Autodesk Inventor part; units mm, degrees
ref_plane "Work Plane1" through (0, 18, 0) normal (0, 1, 0) x (-1, 0, 0)
ref_plane "YZ Plane" through (0, 0, 0) normal (1, 0, 0) x (0, 1, 0)
ref_plane "XY Plane" through (0, 0, 0) normal (0, 0, 1) x (1, 0, 0)
sketch "Sketch1" plane through (0, 0, 0) normal (0, 1, 0) x (-1, 0, 0)
  line L0 (0, 0) -> (80, 0) construction
  line L1 (80, 0) -> (80, 30) construction
  line L2 (80, 30) -> (0, 30) construction
  line L3 (0, 30) -> (0, 0) construction
  dimension "d0" = 80
  dimension "d1" = 30
sketch "Sketch2" plane through (0, 0, 0) normal (0, 1, 0) x (-1, 0, 0)
  line L0 (80, 0) -> (69, 0)
  line L1 (69, 0) -> (69, 30)
  line L2 (69, 30) -> (80, 30)
  line L3 (80, 30) -> (80, 0)
  line L4 (0, 0) -> (11, 0)
  line L5 (11, 0) -> (11, 30)
  line L6 (11, 30) -> (0, 30)
  line L7 (0, 30) -> (0, 0)
  line L8 (57, 0) -> (46, 0)
  line L9 (46, 0) -> (46, 30)
  line L10 (46, 30) -> (57, 30)
  line L11 (57, 30) -> (57, 0)
  line L12 (34, 0) -> (23, 0)
  line L13 (23, 0) -> (23, 30)
  line L14 (23, 30) -> (34, 30)
  line L15 (34, 30) -> (34, 0)
  line L16 (69, 15) -> (57, 15) construction
  line L17 (46, 15) -> (34, 15) construction
  line L18 (23, 15) -> (11, 15) construction
  line L19 (72, 3) -> (77, 3)
  line L20 (77, 3) -> (77, 27)
  line L21 (77, 27) -> (72, 27)
  line L22 (72, 27) -> (72, 3)
  line L23 (54, 3) -> (49, 3)
  line L24 (49, 3) -> (49, 27)
  line L25 (49, 27) -> (54, 27)
  line L26 (54, 27) -> (54, 3)
  line L27 (31, 3) -> (26, 3)
  line L28 (26, 3) -> (26, 27)
  line L29 (26, 27) -> (31, 27)
  line L30 (31, 27) -> (31, 3)
  line L31 (8, 27) -> (8, 3)
  line L32 (8, 3) -> (3, 3)
  line L33 (3, 3) -> (3, 27)
  line L34 (3, 27) -> (8, 27)
  dimension "d2" = 11
  dimension "d3" = 30
  dimension "d4" = 11
  dimension "d6" = 11
  dimension "d8" = 11
  dimension "d9" = 80
  dimension "d10" = 3
  dimension "d11" = 3
  dimension "d12" = 3
  dimension "d13" = 3
extrude "Extrusion1" add sketch "Sketch2" along normal blind 15
sketch "Sketch3" plane through (0, 15, 0) normal (0, 1, 0) x (1, 0, 0)
  line L0 (-69, 0) -> (-80, 0)
  line L1 (-80, 0) -> (-69, 0)
  line L2 (-69, 0) -> (-69, -30)
  line L3 (-69, -30) -> (-80, -30)
  line L4 (-80, -30) -> (-80, 0)
  line L5 (-57, 0) -> (-46, 0)
  line L6 (-46, 0) -> (-46, -30)
  line L7 (-46, -30) -> (-57, -30)
  line L8 (-57, -30) -> (-57, 0)
  line L9 (-34, 0) -> (-23, 0)
  line L10 (-23, 0) -> (-23, -30)
  line L11 (-23, -30) -> (-34, -30)
  line L12 (-34, -30) -> (-34, 0)
  line L13 (-11, 0) -> (0, 0)
  line L14 (0, 0) -> (0, -30)
  line L15 (0, -30) -> (-11, -30)
  line L16 (-11, -30) -> (-11, 0)
  dimension "d16" = 30
  dimension "d19" = 23
extrude "Extrusion2" add sketch "Sketch3" along normal blind 3
sketch "Sketch4" plane through (-69, 0, 30) normal (1, 0, 0) x (0, 0, -1)
  circle A0 centre (7.5, 8) radius 1.5
  line L0 (3, 0) -> (27, 0)
  line L1 (0, 0) -> (0, 18) construction
  dimension "d26" = 3
  dimension "d28" = 8
  dimension "d29" = 7.5
extrude "Extrusion3" cut sketch "Sketch4" against normal blind 3
sketch "Sketch5" plane through (-57, 0, 0) normal (-1, 0, 0) x (0, 0, 1)
  circle A0 centre (22.5, 8) radius 1.5
  line L0 (30, 0) -> (30, 18)
  line L1 (3, 0) -> (27, 0)
  point P0 (0, 0)
  dimension "d33" = 3
  dimension "d34" = 7.5
  dimension "d35" = 8
extrude "Extrusion4" cut sketch "Sketch5" against normal blind 3
sketch "Sketch6" plane through (-46, 0, 30) normal (1, 0, 0) x (0, 0, -1)
  circle A0 centre (22.5, 8) radius 1.5
  line L0 (30, 0) -> (30, 18)
  line L1 (3, 0) -> (27, 0)
  dimension "d38" = 3
  dimension "d39" = 7.5
  dimension "d40" = 8
sketch "Sketch7" plane through (-34, 0, 0) normal (-1, 0, 0) x (0, 0, 1)
  circle A0 centre (7.5, 8) radius 1.5
  line L0 (3, 0) -> (27, 0)
  line L1 (0, 0) -> (0, 18)
  dimension "d41" = 3
  dimension "d42" = 8
  dimension "d43" = 7.5
sketch "Sketch8" plane through (-23, 0, 30) normal (1, 0, 0) x (0, 0, -1)
  circle A0 centre (7.5, 8) radius 1.5
  line L0 (3, 0) -> (27, 0)
  line L1 (0, 0) -> (0, 18)
  point P0 (30, 0)
  dimension "d44" = 3
  dimension "d45" = 8
  dimension "d46" = 7.5
sketch "Sketch9" plane through (-11, 0, 0) normal (-1, 0, 0) x (0, 0, 1)
  point P0 (0, 0)
sketch "Sketch10" plane through (-11, 0, 0) normal (-1, 0, 0) x (0, 0, 1)
  circle A0 centre (22.5, 8) radius 1.5
  line L0 (30, 0) -> (30, 18)
  line L1 (3, 0) -> (27, 0)
  point P0 (0, 0)
  dimension "d47" = 3
  dimension "d48" = 7.5
  dimension "d49" = 8
extrude "Extrusion5" cut sketch "Sketch6" against normal blind 3
extrude "Extrusion6" cut sketch "Sketch7" against normal blind 3
extrude "Extrusion7" cut sketch "Sketch8" against normal blind 3
extrude "Extrusion8" cut sketch "Sketch10" against normal blind 3
ref_plane "Work Plane1" through (0, 18, 0) normal (0, 1, 0) x (-1, 0, 0)
sketch "Sketch12" plane through (0, 18, 0) normal (0, 1, 0) x (-1, 0, 0)
  line L0 (80, 30) -> (50, 30)
  line L1 (50, 30) -> (50, 22)
  line L2 (50, 22) -> (80, 22)
  line L3 (80, 22) -> (80, 30)
  line L4 (55, 0) -> (25, 0)
  line L5 (25, 0) -> (25, 8)
  line L6 (25, 8) -> (55, 8)
  line L7 (55, 8) -> (55, 0)
  line L8 (31, 3) -> (31, 27)
  line L9 (31, 22) -> (1, 22)
  line L10 (1, 22) -> (1, 30)
  line L11 (1, 30) -> (31, 30)
  line L12 (31, 30) -> (31, 22)
  point P0 (0, 0)
  dimension "d59" = 30
  dimension "d60" = 8
  dimension "d61" = 30
  dimension "d62" = 8
  dimension "d63" = 30
sketch "Sketch13" plane through (0, 18, 0) normal (0, 1, 0) x (-1, 0, 0)
  line L0 (74.3573, 0) -> (62.3573, 0)
  line L1 (62.3573, 0) -> (62.3573, 15)
  line L2 (62.3573, 15) -> (74.3573, 15)
  line L3 (74.3573, 15) -> (74.3573, 0)
  line L4 (48, 12) -> (36, 12)
  line L5 (36, 12) -> (36, 21)
  line L6 (36, 21) -> (48, 21)
  line L7 (48, 21) -> (48, 12)
  line L8 (0, 0) -> (11, 0)
  line L9 (4, 0) -> (17, 0)
  line L10 (17, 0) -> (17, 17)
  line L11 (17, 17) -> (4, 17)
  line L12 (4, 17) -> (4, 0)
  dimension "d64" = 12
  dimension "d65" = 15
  dimension "d66" = 12
  dimension "d67" = 13
  dimension "d68" = 17
extrude "Extrusion9" add sketch "Sketch13" along normal blind 2
extrude "Extrusion10" add sketch "Sketch12" along normal blind 4
sketch "Sketch14" plane through (0, 20, 0) normal (0, 1, 0) x (1, 0, 0)
  line L0 (-65, -4) -> (-41.7529, -4)
  line L1 (-41.7529, -4) -> (-41.7529, -17.4715)
  line L2 (-41.7529, -17.4715) -> (-65, -17.4715)
  line L3 (-65, -17.4715) -> (-65, -4)
  line L4 (-12, -25) -> (-28.5, -25)
  line L5 (-28.5, -25) -> (-28.5, -4)
  line L6 (-28.5, -4) -> (-12, -4)
  line L7 (-12, -4) -> (-12, -25)
  point P0 (0, 0)
  dimension "d73" = 16.5
extrude "Extrusion11" add sketch "Sketch14" along normal blind 4
sketch "Sketch15" plane through (0, 20, 0) normal (0, 1, 0) x (1, 0, 0)
  line L0 (-69, -30) -> (-69, -22)
  line L1 (-69, -26) -> (-17, -26)
  line L2 (-17, -26) -> (-17, -6)
  line L3 (-17, -6) -> (-69, -6)
  line L4 (-69, -6) -> (-69, -26)
  point P0 (0, 0)
  dimension "d76" = 52
  dimension "d77" = 20
extrude "Extrusion12" add sketch "Sketch15" along normal blind 3
sketch "Sketch16" plane through (0, 0, 0) normal (0, 1, 0) x (-1, 0, 0)
  line L0 (69, 30) -> (80, 30)
  line L1 (80, 30) -> (80, 36)
  line L2 (69, 30) -> (69, 36)
  line L3 (69, 36) -> (74.8182, 41.4908)
  line L4 (74.8182, 41.4908) -> (80, 36)
  circle A0 centre (74.5, 36) radius 1.25
  line L5 (74.5, 36) -> (80, 36) construction
  line L6 (74.5, 36) -> (69, 36) construction
  line L7 (11, 30) -> (11, 36)
  line L8 (0, 30) -> (0, 36)
  line L9 (11, 36) -> (5.5, 41.8095)
  line L10 (5.5, 41.8095) -> (0, 36)
  circle A1 centre (5.5, 36) radius 1.25
  line L11 (5.5, 36) -> (11, 36) construction
  line L12 (5.5, 36) -> (0, 36) construction
  line L13 (80, 15) -> (0, 15) construction
  line L14 (69, 0) -> (80, 0)
  line L15 (80, 0) -> (80, -6)
  line L16 (69, 0) -> (69, -6)
  line L17 (69, -6) -> (74.8182, -11.4908)
  line L18 (74.8182, -11.4908) -> (80, -6)
  circle A2 centre (74.5, -6) radius 1.25
  line L19 (74.5, -6) -> (80, -6) construction
  line L20 (74.5, -6) -> (69, -6) construction
  line L21 (11, 0) -> (11, -6)
  line L22 (0, 0) -> (0, -6)
  line L23 (11, -6) -> (5.5, -11.8095)
  line L24 (5.5, -11.8095) -> (0, -6)
  circle A3 centre (5.5, -6) radius 1.25
  line L25 (5.5, -6) -> (11, -6) construction
  line L26 (5.5, -6) -> (0, -6) construction
  line L27 (80, 0) -> (69, 0)
  line L28 (80, 0) -> (69, 0)
  line L29 (11, 0) -> (0, 0)
  line L30 (4, 0) -> (17, 0)
  line L31 (11, 30) -> (0, 30)
  dimension "d80" = 6
  dimension "d81" = 6
  dimension "d82" = 8
  dimension "d83" = 2.5
  dimension "d84" = 6
  dimension "d85" = 6
  dimension "d86" = 6
  dimension "d87" = 8
  dimension "d88" = 2.5
extrude "Extrusion14" add sketch "Sketch16" along normal blind 3
equation "\"d84\" = d81"
equation "\"d85\" = d86"
equation "\"d86\" = d84"
equation "\"d87\" = d82"
properties part number "ball-waterfall"
Part model, mm, in its own coordinate system. A direction names the side the tool comes from. Coordinates: 2 decimals unless noted, no trailing zeros. Order: outer loops, then holes, each group sorted by start corner. A loop starts at its lowest first (then second) coordinate and runs counter-clockwise, first axis right, second up. Notation, with made-up numbers: (-11, -2) - (36, -2) arc R31 ccw to (36, 24) - close; hole circle Ø11 at (59.25, 57.5). An arc over 180 degrees is marked (long way). Return JSON: item names as keys, results as strings. Group by question number.
Item 1: Pin check, flat tips, straight feed: pin 1 (12 mm diameter, centred on x = -51.5, z = 26.5, fed in from +Y); pin 2 (4 mm diameter, centred on x = -62, z = 27.5, fed in from -Y); pin 3 (1 mm diameter, centred on x = -12, y = 19, fed in from +Z). Stop position of each tip, or through.
Item 2: Pull direction Y, two halves, no side cores. Call faces 5 (the face through (-71, 0, 15)), 6 (the face through (-24.5, 7.1, 23.7)), 7 (the face through (-77.373, 1.479, 38.784)), 8 (the face through (-70.5, 7.1, 23.7)): pulls with the +Y half, pulls with the -Y half, needs draft (parallel to the pull), parting line crosses it, or undercut.
Item 3: Cut at B-B (y = 8). State how many separate pieces and enclosed holes the cut face has, plus the area to 3 significant figures.
Item 4: Drill centre lines: probe 1 along X at (y, z) = (17, 22); probe 2 along Y at (x, z) = (-55.4, 22.5); probe 3 along Y at (x, z) = (-56.5, 14). Where is each one in solid material? Low to high. Write a range as from..to.
Item 5: Which spindle directions (+Z, -Z, +X, -X, +Y, -Y) get a long thin tool onto all of the face, cutting with end or side? Do faces 1 (the face through (-72, 7, 15)), 2 (the face through (-29, 18, 15)), 3 (the face through (-28.5, 23.4, 14.6)), 4 (the face through (-41, 18, 17)). Say none if no direction does.
Item 6: Cut at A-A (z = -3.5). List the corners of the cut face in (x, y).
Check values:
{
 "1": {"pin 1": "stops at y = 23", "pin 2": "stops at y = 18", "pin 3": "stops at z = 30"},
 "2": {"face 5": "pulls with the -Y half", "face 6": "undercut", "face 7": "needs draft", "face 8": "undercut"},
 "3": {"separate pieces": "6", "enclosed holes": "0", "area": "786 mm2"},
 "4": {"probe 1": "x = -80..-69, -57..-46, -34..-23, -11..0", "probe 2": "y = 0..6.5, 9.5..23", "probe 3": "y = 0..18, 20..24"},
 "5": {"face 1": "-Y", "face 2": "none", "face 3": "-Z, +Y", "face 4": "+Z, -Z, -Y"},
 "6": {"outline": "(-80, 0) - (-69, 0) - (-69, 3) - (-80, 3) - close; (-11, 0) - (0, 0) - (0, 3) - (-11, 3) - close"}
}
